The listing builds one solid part. Answer for the finished solid, in the listing's coordinates (mm). A direction names the side the tool comes from. Give positions to 0.01 mm unless a question says otherwise; leave off trailing zeros. Order: outer loops, then holes, each group sorted by start corner. A loop starts at its lowest first (then second) coordinate and runs counter-clockwise, first axis right, second up. Notation, with made-up numbers: (-4.75, -11.5) - (9.25, -11.5) arc R11 cw to (9.25, 3.5) - close; hole circle Ø1 at (64, 50.25). An arc over 180 degrees is marked (long way). Write each question's results on one line, items separated by ' | '. Start each with the question number.
1. Find the intervals of material crossed by L1, parallel to Y at x = 0, z = 1.65; L2, parallel to Z at x = 8, y = 4; L3, parallel to X at y = 4.5, z = 1.85, in increasing order.
2. Section C-C (z = 2.6) is taken. Give the vertices of the cut face in (x, y), and give its area (3 significant figures).
3. Determine the mould class of faces 3 (the face through (4, -4, 0)), 4 (the face through (-6, 0, 2)), 5 (the face through (-1.08, 4.88, 1.97)) for opening direction Y: released by +Y, released by -Y, zero draft, split by the parting line, or undercut.
4. Which of the six approach directions +Z, -Z, +X, -X, +Y, -Y give full straight-line access (tool end or side, diameter ignored) to faces 1 (the face through (2, -6, 1)), 2 (the face through (-1.172, -8.923, 0.493))?
5. Section D-D (x = 7.75) is taken. Give the vertices of the cut face in (y, z).
6. Section A-A (y = 0) is taken. Give the vertices of the cut face in (x, z).
7. Flat-ended cylindrical pins translate along their axes: pin 1 (1 mm diameter, centred on x = 4.5, y = 3.5, fed in from +Z); pin 2 (1 mm diameter, centred on x = -3, y = -7, fed in from +Z). Find the tip coordinate at first contact, or state that the pin passes through.
Autodesk Inventor part; units mm, degrees
ref_plane "YZ Plane" through (0, 0, 0) normal (1, 0, 0) x (0, 1, 0)
ref_plane "XZ Plane" through (0, 0, 0) normal (0, 1, 0) x (-1, 0, 0)
ref_plane "XY Plane" through (0, 0, 0) normal (0, 0, 1) x (1, 0, 0)
sketch "スケッチ1" plane through (0, 0, 0) normal (0, 0, 1) x (1, 0, 0)
  circle A0 centre (0, 0) radius 5
  circle A1 centre (0, 0) radius 9
  dimension "d0" = 10
  dimension "d1" = 18
extrude "押し出し1" add sketch "スケッチ1" along normal blind 1
sketch "スケッチ2" plane through (0, 0, 1) normal (0, 0, 1) x (1, 0, 0)
  circle A0 centre (0, 0) radius 6
  circle A1 centre (0, 0) radius 9
  circle A2 centre (0, 0) radius 5
  dimension "d4" = 12
extrude "押し出し2" add sketch "スケッチ2" along normal blind 3 contours A0
chamfer "面取り1" distance 0.5 angle 45 1 edges at (-6, 0, 4)
properties part number "オイレスw5f10-12a" material "アセタール樹脂、黒"
Reported:
1) L1: -6 to -5, 5 to 6 | L2: 0 to 1 | L3: -3.97 to -2.18, 2.18 to 3.97
2) outline: circle Ø12 at (0, 0); hole circle Ø10 at (0, 0) | area: 34.6 mm²
3) face 3: zero draft | face 4: split by the parting line | face 5: undercut
4) face 1: +Z | face 2: +Z, -Z
5) outline: (-4.58, 0) - (4.58, 0) - (4.58, 1) - (-4.58, 1) - close
6) outline: (-9, 0) - (-5, 0) - (-5, 4) - (-5.5, 4) - (-6, 3.5) - (-6, 1) - (-9, 1) - close; (5, 0) - (9, 0) - (9, 1) - (6, 1) - (6, 3.5) - (5.5, 4) - (5, 4) - close
7) pin 1: z = 4 | pin 2: z = 1
